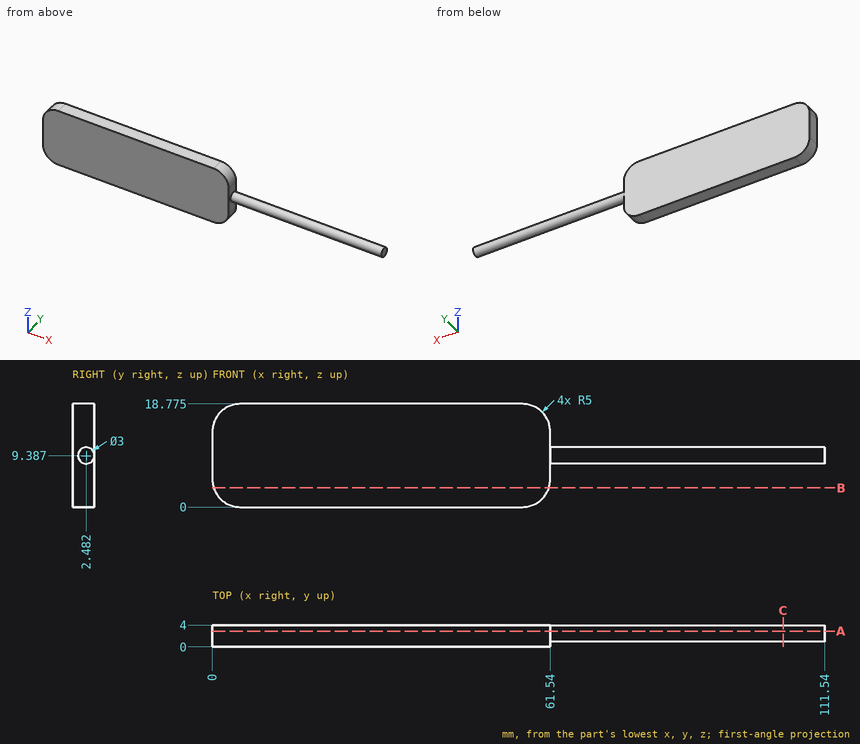
Design review of the part shown in the three views and the two pictorial views. Dimensions are in mm from the part's minimum x, y and z. Coordinates: 2 decimals unless noted, no trailing zeros. Write each loop counter-clockwise with the first axis right and the second up, starting at its lowest first coordinate (ties: lowest second). Pieces come first, ordered by that corner, then holes.
1) Clearance check with flat-ended pins moving along their axes: pin 1 Ø1.5 at (x, z) = (82, 11) entering from +Y; pin 2 Ø2 at (y, z) = (1, 3.5) entering from -X (1 decimal). State where each tip first meets the part, or that it passes through.
2) We need section B-B on z = 3.5. State the section outline as (x, y) points.
3) To check wall thickness, follow probe 1 along X at (y, z) = (1.35, 4.75); probe 2 along X at (y, z) = (1.75, 14.5); probe 3 along Z at (x, y) = (73, 3.85) (1 decimal). State the ranges of each line that lie inside material, in increasing order.
4) We need section A-A on y = 2.9. State the section outline as (x, z) points (1 decimal), then the cut area to 3 significant figures.
5) We need section C-C on x = 104. State the section outline as (y, z) points.
Answer list:
1. pin 1: stops at y = 3.71
1. pin 2: stops at x = 0
2. outline: (0.23, 0) - (61.31, 0) - (61.31, 4) - (0.23, 4) - close
3. probe 1: x = 0.01 to 61.53
3. probe 2: x = 0.05 to 61.49
3. probe 3: z = 8.8 to 10
4. outline: (0, 5) arc R5 ccw to (5, 0) - (56.5, 0) arc R5 ccw to (61.5, 5) - (61.5, 7.9) - (111.5, 7.9) - (111.5, 10.8) - (61.5, 10.8) - (61.5, 13.8) arc R5 ccw to (56.5, 18.8) - (5, 18.8) arc R5 ccw to (0, 13.8) - close
4. area: 1,280 mm2
5. outline: circle Ø3 at (2.48, 9.39)
